```python
from build123d import *

# Parameters (mm, degrees)
F0_W     = 498
F0_H     = 774
F1_DEPTH = 25
F2_W     = 398
F2_H     = 674
F3_DEPTH = 15
F5_DEPTH = 25
F6_W     = 30
F6_H     = 80
F7_DEPTH = 5


with BuildPart() as f1:
    # F0 (on Front) → F1 (new body)
    with BuildSketch(Plane.XZ):
        Rectangle(F0_W, F0_H)
    extrude(amount=F1_DEPTH)

    # F2 (on face) → F3 (cut)
    with BuildSketch(Plane.XZ.offset(25)):
        Rectangle(F2_W, F2_H)
    extrude(amount=-F3_DEPTH, mode=Mode.SUBTRACT)

    # F4 (on face) → F5 (cut, through all)
    with BuildSketch(Plane.XZ.offset(25)):
        with BuildLine():
            ThreePointArc((228, 255), (221.171573, 257.828427), (224, 251))
            ThreePointArc((224, 251), (226.828427, 252.171573), (228, 255))
        make_face()
        with BuildLine():
            ThreePointArc((228, 145), (226.828427, 147.828427), (224, 149))
            ThreePointArc((224, 149), (221.171573, 142.171573), (228, 145))
        make_face()
    extrude(amount=-F5_DEPTH, mode=Mode.SUBTRACT)

    # F6 (on face) → F7 (cut)
    with BuildSketch(Plane(origin=(0, 0, 0), x_dir=(-1, 0, 0), z_dir=(0, 1, 0))):
        with Locations((209, 317)):
            Rectangle(F6_W, F6_H)
        with Locations((209, -317)):
            Rectangle(F6_W, F6_H)
    extrude(amount=-F7_DEPTH, mode=Mode.SUBTRACT)


solid = f1.part
```
Here's how the part is built. I have some questions about the finished solid (model axes, mm). A direction names the side the tool comes from. Give positions to 0.01 mm unless a question says otherwise; leave off trailing zeros. Loops run counter-clockwise (first coordinate to the right, second up) from the corner with the lowest first, then second, coordinate; pieces in that order, holes last. Notation, with made-up numbers: M -28,48.5 L 21,48.5 A15 ccw 21,56.5 Z; hole C 34.5,82 d5. An arc over 180 degrees is marked long. Return JSON: item names as keys, results as strings.
Item 1: I'm going to push flat-ended pins straight in: pin 1 Ø12 at (x, z) = (-151.5, 90) entering from -Y; pin 2 Ø8 at (x, z) = (112.5, -273.5) entering from +Y; pin 3 Ø9 at (x, z) = (-211, 309) entering from +Y. Where does each tip first touch, or does it pass through?
A:
{"pin 1": "stops at y = -10", "pin 2": "stops at y = 0", "pin 3": "stops at y = -5"}
Item 2: Imagine slicing it at B-B on z = -51. List the corners of the cut face in (x, y) for me.
A:
{"outline": "M -249,-25 L -199,-25 L -199,-10 L 199,-10 L 199,-25 L 249,-25 L 249,0 L -249,0 Z"}
Item 3: Imagine slicing it at C-C on x = -88. List the corners of the cut face in (y, z) for me.
A:
{"outline": "M -25,-387 L 0,-387 L 0,387 L -25,387 L -25,337 L -10,337 L -10,-337 L -25,-337 Z"}
Item 4: On a 3-axis mill with a long thin cutter (end or side, diameter ignored), from which of +Z, -Z, +X, -X, +Y, -Y can I reach the whole of each face in a straight line? I mean faces 1 (the flat face through (-209, -5, 318)), 2 (the flat face through (-3, -12, -387)), 3 (the flat face through (-199, -18, -5)). Say none if no direction works.
A:
{"face 1": "+Y", "face 2": "-Z, +X, -X, +Y, -Y", "face 3": "-Y"}
Item 5: Please list where these lines run through material, in increasing order: line 1 (X direction, y = -19.5, z = 255); line 2 (Z direction, x = 224, y = -14.75); line 3 (X direction, y = -9.25, z = 145).
A:
{"line 1": "x = -249 to -199, 199 to 220, 228 to 249", "line 2": "z = -387 to 141, 149 to 251, 259 to 387", "line 3": "x = -249 to 220, 228 to 249"}
Item 6: Imagine slicing it at D-D on z = 318. List the corners of the cut face in (x, y) for me, then the cut area to 3 significant figures.
A:
{"outline": "M -249,-25 L -199,-25 L -199,-10 L 199,-10 L 199,-25 L 249,-25 L 249,0 L -194,0 L -194,-5 L -224,-5 L -224,0 L -249,0 Z", "area": "6,330 mm^2"}
Item 7: Thinking about a two-plate mould opening in Z: for faces 4 (the flat face through (-3, -18, 337)), 5 (the flat face through (-249, -12, -5)), 6 (the flat face through (-3, -12, 387)), which applies, released by +Z, released by -Z, zero draft, split by the parting line, or undercut?
A:
{"face 4": "undercut", "face 5": "zero draft", "face 6": "released by +Z"}
Item 8: Imagine slicing it at A-A on y = -20.75. List the corners of the cut face in (x, z) for me.
A:
{"outline": "M -249,-387 L 249,-387 L 249,387 L -249,387 Z; hole M -199,-337 L 199,-337 L 199,337 L -199,337 Z; hole C 224,145 d8; hole C 224,255 d8"}
